Autodesk Inventor part; units mm, degrees
ref_plane "YZ Plane" through (0, 0, 0) normal (1, 0, 0) x (0, 1, 0)
ref_plane "XZ Plane" through (0, 0, 0) normal (0, 1, 0) x (-1, 0, 0)
ref_plane "XY Plane" through (0, 0, 0) normal (0, 0, 1) x (1, 0, 0)
sketch "Sketch1" plane through (0, 0, 0) normal (0, 1, 0) x (-1, 0, 0)
  line L0 (22.5, 13) -> (-22.5, 13)
  line L1 (-22.5, 13) -> (-22.5, -13)
  line L2 (-22.5, -13) -> (22.5, -13)
  line L3 (22.5, -13) -> (22.5, 13)
  line L4 (13, 23) -> (-13, 23)
  line L5 (-13, 23) -> (-13, -23)
  line L6 (-13, -23) -> (13, -23)
  line L7 (13, -23) -> (13, 23)
  line L8 (13, -23) -> (-13, 23) construction
  line L9 (13, 23) -> (-13, -23) construction
  line L10 (22.5, -13) -> (-22.5, 13) construction
  line L11 (22.5, 13) -> (-22.5, -13) construction
  line L12 (13, -23) -> (-13, -23)
  line L13 (-13, -23) -> (-13, -20)
  line L14 (-13, -20) -> (13, -20)
  line L15 (13, -20) -> (13, -23)
  line L16 (13, 23) -> (-13, 23)
  line L17 (-13, 23) -> (-13, 20)
  line L18 (-13, 20) -> (13, 20)
  line L19 (13, 20) -> (13, 23)
  line L20 (22.5, 13) -> (19.5, 13)
  line L21 (19.5, 13) -> (19.5, -13)
  line L22 (19.5, -13) -> (22.5, -13)
  line L23 (22.5, -13) -> (22.5, 13)
  line L24 (-22.5, 13) -> (-19.5, 13)
  line L25 (-19.5, 13) -> (-19.5, -13)
  line L26 (-19.5, -13) -> (-22.5, -13)
  line L27 (-22.5, -13) -> (-22.5, 13)
  point P0 (0, 0)
  point P1 (0, 0)
  point P2 (0, 0)
  point P3 (-19.5, 13)
  point P4 (13, 20)
  point P5 (13, 13)
  point P6 (-13, 13)
  point P7 (-13, -13)
  point P8 (13, -13)
  dimension "d0" = 45
  dimension "d1" = 46
  dimension "d2" = 26
  dimension "d3" = 26
  dimension "d4" = 3
  dimension "d5" = 3
  dimension "d6" = 3
  dimension "d7" = 3
extrude "Extrusion1" add sketch "Sketch1" along normal blind 28 contours L3 L2 L21 L0 | L25 L2 L1 L0
extrude "Extrusion2" add sketch "Sketch1" against normal blind 30 contours L18 L5 L4 L7 | L7 L6 L5 L14
extrude "Extrusion3" add sketch "Sketch1" along normal mid plane 4 contours L21 L2 L7 L0 | L7 L2 L5 L0 | L0 L5 L18 L7 | L5 L2 L25 L0 | L7 L14 L5 L2
extrude "Extrusion4" add sketch "Sketch1" along normal blind 2 contours L18 L5 L4 L7 | L7 L6 L5 L14
extrude "Extrusion5" add sketch "Sketch1" against normal blind 2 contours L3 L2 L21 L0 | L25 L2 L1 L0
sketch "Sketch2" plane through (22.5, 28, 13) normal (1, 0, 0) x (0, 0, -1)
  line L0 (0, 0) -> (26, 0)
  line L1 (13, 0) -> (13, -11.5)
  circle A0 centre (21, -11.5) radius 1
  circle A1 centre (5, -11.5) radius 1
  point P0 (13, -28)
  dimension "d18" = 11.5
  dimension "d73" = 2
  dimension "d74" = 8
extrude "Extrusion6" cut sketch "Sketch2" against normal blind 60
sketch "Sketch6" plane through (22.5, 28, 13) normal (1, 0, 0) x (0, 0, -1)
  line L0 (0, 0) -> (26, 0)
  line L1 (8, 0) -> (0, -8)
  line L2 (0, -30) -> (0, 0)
  line L3 (18, 0) -> (26, -8)
  line L4 (26, -26) -> (26, 0)
  point P0 (13, -28)
  dimension "d43" = 8
  dimension "d44" = 8
  dimension "d45" = 8
  dimension "d46" = 8
extrude "Extrusion9" cut sketch "Sketch6" against normal blind 50
sketch "Sketch7" plane through (-13, -30, 23) normal (0, 0, 1) x (1, 0, 0)
  line L0 (0, 28) -> (0, 0)
  line L1 (0, 8) -> (8, 0)
  line L2 (0, 0) -> (26, 0)
  line L3 (26, 0) -> (26, 8)
  line L4 (26, 8) -> (18, 0)
  point P0 (13, 30)
  dimension "d49" = 8
  dimension "d50" = 8
  dimension "d51" = 8
  dimension "d52" = 8
extrude "Extrusion10" cut sketch "Sketch7" against normal blind 50
sketch "Sketch9" plane through (13, 2, -23) normal (0, 0, -1) x (-1, 0, 0)
  line L0 (18, -32) -> (8, -32)
  line L1 (13, -32) -> (13, -20.5)
  line L2 (13, -32) -> (24.5, -32) construction
  circle A0 centre (13, -12.5) radius 1
  circle A1 centre (5, -20.5) radius 1
  circle A2 centre (13, -28.5) radius 1
  circle A3 centre (21, -20.5) radius 1
  point P0 (13, -2)
  dimension "d59" = 11.5
  dimension "d60" = 90
  dimension "d61" = 2
  dimension "d62" = 8
  dimension "d65" = 360
extrude "Extrusion12" cut sketch "Sketch9" against normal blind 3
sketch "Sketch10" plane through (-13, 2, 23) normal (0, 0, 1) x (1, 0, 0)
  line L0 (18, -32) -> (8, -32)
  line L1 (13, -32) -> (13, -20.5)
  circle A0 centre (13, -20.5) radius 1.5
  point P0 (13, -2)
  dimension "d69" = 11.5
  dimension "d70" = 3
extrude "Extrusion13" cut sketch "Sketch10" against normal blind 3
properties part number "first_junction"
CAD build for the part. Positions are in the model's coordinates, mm. A direction names the side the tool comes from. Coordinates: 2 decimals unless noted, no trailing zeros. Write each loop counter-clockwise with the first axis right and the second up, starting at its lowest first coordinate (ties: lowest second). Pieces come first, ordered by that corner, then holes. Notation, with made-up numbers: M 24.5,65.5 L 61.5,65.5 A20 cw 61.5,92.5 Z; hole C 87.25,34 d1. An arc over 180 degrees is marked long. Answer as a JSON object with one key per item and string values. Group by question number.
1) Wall check: line 1 (X direction, y = 4.5, z = 9.5); line 2 (Z direction, x = 2.5, y = -21.5); line 3 (Y direction, x = 0, z = 21.2). Give the ranges that are in metal, low to high. Write a range as from..to.
2) Saw through at D-D (y = -26.5). Write the cut outline in (x, z), plus the area to 3 significant figures.
3) Pin check, flat tips, straight feed: pin 1 Ø8 at (y, z) = (-4.5, -17.5) entering from +X; pin 2 Ø2.5 at (x, y) = (0, -18.5) entering from +Z; pin 3 Ø3 at (x, z) = (1, -11) entering from +Y; pin 4 Ø3 at (x, y) = (0, -10.5) entering from -Z. Stop position of each tip, or through.
4) Mould opens along Z. For faces 1 (the face through (-9, -26, -21)), 2 (the face through (0, -14, -23)), 3 (the face through (21.021, 15.524, 8.217)), 4 (the face through (21, 24, 9)) say: +Z half, -Z half, draft (parallel to the pull), parting line (faces both ways), or undercut.
5) Saw through at A-A (y = 24.5). Write the cut outline in (x, z).
6) Tool access for faces 5 (the face through (0.13, -9.51, -21.52)), 6 (the face through (-20, 6, -13)), 7 (the face through (0, -16, 20)), 8 (the face through (0, 2, 0)): list every direction of +Z, -Z, +X, -X, +Y, -Y with a clear straight run to the whole face (end or side of a thin tool).
7) Saw through at C-C (z = 8). Write the cut outline in (x, y), plus the area to 3 significant figures.
8) Saw through at B-B (x = 8). Write the cut outline in (y, z).
Values follow:
{
 "1": {"line 1": "x = -22.5..-19.5, 19.5..22.5", "line 2": "z = -23..-20, 20..23", "line 3": "y = -30..-20, -17..2"},
 "2": {"outline": "M -8.5,-23 L -1,-23 L -1,-20 L -8.5,-20 Z; M -8.5,20 L 8.5,20 L 8.5,23 L -8.5,23 Z; M 1,-23 L 8.5,-23 L 8.5,-20 L 1,-20 Z", "area": "96.0 mm2"},
 "3": {"pin 1": "stops at x = 13", "pin 2": "stops at z = -20", "pin 3": "stops at y = 2", "pin 4": "stops at z = -23"},
 "4": {"face 1": "draft", "face 2": "-Z half", "face 3": "undercut", "face 4": "+Z half"},
 "5": {"outline": "M -22.5,-8.5 L -19.5,-8.5 L -19.5,8.5 L -22.5,8.5 Z; M 19.5,-8.5 L 22.5,-8.5 L 22.5,8.5 L 19.5,8.5 Z"},
 "6": {"face 5": "-Z", "face 6": "-Z, -X, +Y, -Y", "face 7": "+X, -X, -Y", "face 8": "+Z, -Z, +Y"},
 "7": {"outline": "M -22.5,-2 L 22.5,-2 L 22.5,15.5 L 19.5,15.5 L 19.5,2 L -19.5,2 L -19.5,15.5 L -22.5,15.5 Z; M -22.5,17.5 L -19.5,17.5 L -19.5,25 L -22.5,25 Z; M 19.5,17.5 L 22.5,17.5 L 22.5,25 L 19.5,25 Z", "area": "306 mm2"},
 "8": {"outline": "M -27,-23 L -19.5,-23 L -19.5,-20 L -27,-20 Z; M -27,20 L -2,20 L -2,-20 L -17.5,-20 L -17.5,-23 L 2,-23 L 2,23 L -27,23 Z"}
}
